```python
from build123d import *

# Parameters (mm, degrees)
F1_DEPTH = 4
F2_R     = 2.5
F3_DEPTH = 4.001


with BuildPart() as f1:
    # F0 (on Right) → F1 (new body)
    with BuildSketch(Plane.YZ):
        with BuildLine():
            ThreePointArc((0.186993, 10.007145), (0, 10.136198), (-0.186993, 10.007145))
            Line((-0.186993, 10.007145), (-1.049264, 7.734473))
            ThreePointArc((-1.049264, 7.734473), (-1.20497, 7.607883), (-1.392175, 7.680162))
            Line((-1.392175, 7.680162), (-2.914536, 9.575144))
            ThreePointArc((-2.914536, 9.575144), (-3.132257, 9.640097), (-3.270219, 9.459576))
            Line((-3.270219, 9.459576), (-3.387993, 7.031681))
            ThreePointArc((-3.387993, 7.031681), (-3.49696, 6.86317), (-3.697337, 6.874062))
            Line((-3.697337, 6.874062), (-5.730771, 8.205862))
            ThreePointArc((-5.730771, 8.205862), (-5.957908, 8.200356), (-6.033333, 7.986038))
            Line((-6.033333, 7.986038), (-5.395082, 5.640579))
            ThreePointArc((-5.395082, 5.640579), (-5.446643, 5.446643), (-5.640579, 5.395082))
            Line((-5.640579, 5.395082), (-7.986038, 6.033333))
            ThreePointArc((-7.986038, 6.033333), (-8.200356, 5.957908), (-8.205862, 5.730771))
            Line((-8.205862, 5.730771), (-6.874062, 3.697337))
            ThreePointArc((-6.874062, 3.697337), (-6.86317, 3.49696), (-7.031681, 3.387993))
            Line((-7.031681, 3.387993), (-9.459576, 3.270219))
            ThreePointArc((-9.459576, 3.270219), (-9.640097, 3.132257), (-9.575144, 2.914536))
            Line((-9.575144, 2.914536), (-7.680162, 1.392175))
            ThreePointArc((-7.680162, 1.392175), (-7.607883, 1.20497), (-7.734473, 1.049264))
            Line((-7.734473, 1.049264), (-10.007145, 0.186993))
            ThreePointArc((-10.007145, 0.186993), (-10.136198, 0), (-10.007145, -0.186993))
            Line((-10.007145, -0.186993), (-7.734473, -1.049264))
            ThreePointArc((-7.734473, -1.049264), (-7.607883, -1.20497), (-7.680162, -1.392175))
            Line((-7.680162, -1.392175), (-9.575144, -2.914536))
            ThreePointArc((-9.575144, -2.914536), (-9.640097, -3.132257), (-9.459576, -3.270219))
            Line((-9.459576, -3.270219), (-7.031681, -3.387993))
            ThreePointArc((-7.031681, -3.387993), (-6.86317, -3.49696), (-6.874062, -3.697337))
            Line((-6.874062, -3.697337), (-8.205862, -5.730771))
            ThreePointArc((-8.205862, -5.730771), (-8.200356, -5.957908), (-7.986038, -6.033333))
            Line((-7.986038, -6.033333), (-5.640579, -5.395082))
            ThreePointArc((-5.640579, -5.395082), (-5.446643, -5.446643), (-5.395082, -5.640579))
            Line((-5.395082, -5.640579), (-6.033333, -7.986038))
            ThreePointArc((-6.033333, -7.986038), (-5.957908, -8.200356), (-5.730771, -8.205862))
            Line((-5.730771, -8.205862), (-3.697337, -6.874062))
            ThreePointArc((-3.697337, -6.874062), (-3.49696, -6.86317), (-3.387993, -7.031681))
            Line((-3.387993, -7.031681), (-3.270219, -9.459576))
            ThreePointArc((-3.270219, -9.459576), (-3.132257, -9.640097), (-2.914536, -9.575144))
            Line((-2.914536, -9.575144), (-1.392175, -7.680162))
            ThreePointArc((-1.392175, -7.680162), (-1.20497, -7.607883), (-1.049264, -7.734473))
            Line((-1.049264, -7.734473), (-0.186993, -10.007145))
            ThreePointArc((-0.186993, -10.007145), (0, -10.136198), (0.186993, -10.007145))
            Line((0.186993, -10.007145), (1.049264, -7.734473))
            ThreePointArc((1.049264, -7.734473), (1.20497, -7.607883), (1.392175, -7.680162))
            Line((1.392175, -7.680162), (2.914536, -9.575144))
            ThreePointArc((2.914536, -9.575144), (3.132257, -9.640097), (3.270219, -9.459576))
            Line((3.270219, -9.459576), (3.387993, -7.031681))
            ThreePointArc((3.387993, -7.031681), (3.49696, -6.86317), (3.697337, -6.874062))
            Line((3.697337, -6.874062), (5.730771, -8.205862))
            ThreePointArc((5.730771, -8.205862), (5.957908, -8.200356), (6.033333, -7.986038))
            Line((6.033333, -7.986038), (5.395082, -5.640579))
            ThreePointArc((5.395082, -5.640579), (5.446643, -5.446643), (5.640579, -5.395082))
            Line((5.640579, -5.395082), (7.986038, -6.033333))
            ThreePointArc((7.986038, -6.033333), (8.200356, -5.957908), (8.205862, -5.730771))
            Line((8.205862, -5.730771), (6.874062, -3.697337))
            ThreePointArc((6.874062, -3.697337), (6.86317, -3.49696), (7.031681, -3.387993))
            Line((7.031681, -3.387993), (9.459576, -3.270219))
            ThreePointArc((9.459576, -3.270219), (9.640097, -3.132257), (9.575144, -2.914536))
            Line((9.575144, -2.914536), (7.680162, -1.392175))
            ThreePointArc((7.680162, -1.392175), (7.607883, -1.20497), (7.734473, -1.049264))
            Line((7.734473, -1.049264), (10.007145, -0.186993))
            ThreePointArc((10.007145, -0.186993), (10.136198, 0), (10.007145, 0.186993))
            Line((10.007145, 0.186993), (7.734473, 1.049264))
            ThreePointArc((7.734473, 1.049264), (7.607883, 1.20497), (7.680162, 1.392175))
            Line((7.680162, 1.392175), (9.575144, 2.914536))
            ThreePointArc((9.575144, 2.914536), (9.640097, 3.132257), (9.459576, 3.270219))
            Line((9.459576, 3.270219), (7.031681, 3.387993))
            ThreePointArc((7.031681, 3.387993), (6.86317, 3.49696), (6.874062, 3.697337))
            Line((6.874062, 3.697337), (8.205862, 5.730771))
            ThreePointArc((8.205862, 5.730771), (8.200356, 5.957908), (7.986038, 6.033333))
            Line((7.986038, 6.033333), (5.640579, 5.395082))
            ThreePointArc((5.640579, 5.395082), (5.446643, 5.446643), (5.395082, 5.640579))
            Line((5.395082, 5.640579), (6.033333, 7.986038))
            ThreePointArc((6.033333, 7.986038), (5.957908, 8.200356), (5.730771, 8.205862))
            Line((5.730771, 8.205862), (3.697337, 6.874062))
            ThreePointArc((3.697337, 6.874062), (3.49696, 6.86317), (3.387993, 7.031681))
            Line((3.387993, 7.031681), (3.270219, 9.459576))
            ThreePointArc((3.270219, 9.459576), (3.132257, 9.640097), (2.914536, 9.575144))
            Line((2.914536, 9.575144), (1.392175, 7.680162))
            ThreePointArc((1.392175, 7.680162), (1.20497, 7.607883), (1.049264, 7.734473))
            Line((1.049264, 7.734473), (0.186993, 10.007145))
        make_face()
    extrude(amount=F1_DEPTH)

    # F2 (on Right) → F3 (cut, through all)
    with BuildSketch(Plane.YZ):
        Circle(F2_R)
    extrude(amount=F3_DEPTH, mode=Mode.SUBTRACT)


solid = f1.part
```
Read the model definition and answer for the solid it produces. Units are mm, in the model's axes. A direction names the side the tool comes from. Give positions to 0.01 mm unless a question says otherwise; leave off trailing zeros. Order: outer loops, then holes, each group sorted by start corner. A loop starts at its lowest first (then second) coordinate and runs counter-clockwise, first axis right, second up.
(1) Find section A-A (y = -0.75). Give the vertices of the cut face in (x, z), plus the area to 3 significant figures.
(2) Straight lines are drawn through the part: L1, parallel to Y at x = 2.35, z = 0; L2, parallel to Y at x = 0.95, z = 9. For each, find the intervals that lie inside material, in ascending order.
(3) Find section B-B (z = -4.25). Give the vertices of the cut face in (x, y).
(4) For faces 4 (the flat face through (1.972, 0.624, 8.855)), 5 (the flat face through (1.97, 2.14, -8.61)), 6 (the flat face through (1.972, 8.855, -0.624)), determine the directions among +Z, -Z, +X, -X, +Y, -Y from which every point of the face is accessible in a straight line to the end or side of a thin tool.
(5) Find section C-C (y = -5). Give the vertices of the cut face in (x, z), plus the area to 3 significant figures.
(6) For a pull along Y with two mould halves and no side action, classify faces 1 (the flat face through (1.97, 7.53, 4.7)), 2 (the flat face through (1.97, 4.73, 7.55)), 3 (the flat face through (1.97, -8.26, -3.33)) as released by +Y, released by -Y, zero draft, split by the parting line, or undercut.
(7) Given pin 1 (1.5 mm diameter, centred on x = 1.5, z = 6, fed in from -Y); pin 2 (2 mm diameter, centred on x = 3, y = 6.5, fed in from -Z), each flat-ended and moving along its own axis, determine where each tip first touches the part or whether it passes through.
Result sheet:
1. outline: (0, -8.52) - (4, -8.52) - (4, -2.38) - (0, -2.38) - close; (0, 2.38) - (4, 2.38) - (4, 8.52) - (0, 8.52) - close
1. area: 49.1 mm2
2. L1: y = -10.14 to -2.5, 2.5 to 10.14
2. L2: y = -3.29 to -2.45, -0.57 to 0.57, 2.45 to 3.29
3. outline: (0, -7.24) - (4, -7.24) - (4, 7.24) - (0, 7.24) - close
4. face 4: +Z, +X, -X
4. face 5: -Z, +X, -X
4. face 6: +X, -X, +Y
5. outline: (0, -7.73) - (4, -7.73) - (4, 7.73) - (0, 7.73) - close
5. area: 61.8 mm2
6. face 1: released by +Y
6. face 2: undercut
6. face 3: released by -Y
7. pin 1: stops at y = -8.24
7. pin 2: stops at z = -8.24
